from build123d import *

# Parameters (mm, degrees)
BOSS_EXTRUDE1_DEPTH = 0.7366
BOSS_EXTRUDE2_START = 5.3848
BOSS_EXTRUDE2_DEPTH = 0.7366
SKETCH2_R           = 1.1557
BOSS_EXTRUDE3_DEPTH = 4.6482
BOSS_EXTRUDE4_START = -5.3848
BOSS_EXTRUDE4_DEPTH = 0.7366
BOSS_EXTRUDE5_START = -6.1214
SKETCH2_2_R         = 1.1557
BOSS_EXTRUDE5_DEPTH = 4.6482


with BuildPart() as part:
    # Sketch1 → Boss-Extrude1 (new, symmetric)
    with BuildSketch(Plane.XY):
        with BuildLine():
            ThreePointArc((-1.5875, 2.421640582), (-6.0706, 0), (-1.5875, -2.421640582))
            ThreePointArc((-1.5875, -2.421640582), (0, -1.947681165), (1.5875, -2.421640582))
            ThreePointArc((1.5875, -2.421640582), (6.0706, 0), (1.5875, 2.421640582))
            ThreePointArc((1.5875, 2.421640582), (0, 1.947681165), (-1.5875, 2.421640582))
        make_face()
    extrude(amount=BOSS_EXTRUDE1_DEPTH, both=True)



with BuildPart() as body_2:
    # Sketch1<2> → Boss-Extrude2 (new body)
    with BuildSketch(Plane.XY.offset(BOSS_EXTRUDE2_START)):
        with BuildLine():
            ThreePointArc((-1.5875, 2.421640582), (-6.0706, 0), (-1.5875, -2.421640582))
            ThreePointArc((-1.5875, -2.421640582), (0, -1.947681165), (1.5875, -2.421640582))
            ThreePointArc((1.5875, -2.421640582), (6.0706, 0), (1.5875, 2.421640582))
            ThreePointArc((1.5875, 2.421640582), (0, 1.947681165), (-1.5875, 2.421640582))
        make_face()
    extrude(amount=BOSS_EXTRUDE2_DEPTH)


with BuildPart() as part_1:
    add(part.part)

    add(body_2.part)  # Boss-Extrude3 merges body 2
    # Sketch2 → Boss-Extrude3 (add)
    with BuildSketch(Plane.XY.offset(0.7366)):
        with Locations((-3.175, 0)):
            Circle(SKETCH2_R)
        with Locations((3.175, 0)):
            Circle(SKETCH2_R)
    extrude(amount=BOSS_EXTRUDE3_DEPTH)



with BuildPart() as body_2_2:
    # Sketch1<3> → Boss-Extrude4 (new body)
    with BuildSketch(Plane.XY.offset(BOSS_EXTRUDE4_START)):
        with BuildLine():
            ThreePointArc((-1.5875, 2.421640582), (-6.0706, 0), (-1.5875, -2.421640582))
            ThreePointArc((-1.5875, -2.421640582), (0, -1.947681165), (1.5875, -2.421640582))
            ThreePointArc((1.5875, -2.421640582), (6.0706, 0), (1.5875, 2.421640582))
            ThreePointArc((1.5875, 2.421640582), (0, 1.947681165), (-1.5875, 2.421640582))
        make_face()
    extrude(amount=-BOSS_EXTRUDE4_DEPTH)


with BuildPart() as part_2:
    add(part_1.part)

    add(body_2_2.part)  # Boss-Extrude5 merges body 2 2
    # Sketch2<2> → Boss-Extrude5 (add)
    with BuildSketch(Plane.XY.offset(0.7366).offset(BOSS_EXTRUDE5_START)):
        with Locations((-3.175, 0)):
            Circle(SKETCH2_2_R)
        with Locations((3.175, 0)):
            Circle(SKETCH2_2_R)
    extrude(amount=BOSS_EXTRUDE5_DEPTH)


solid = part_2.part
For this review, take the finished solid that the model builds, in its own axes (mm). A direction names the side the tool comes from. Round coordinates to 2 decimals unless told otherwise and drop trailing zeros. Loops run counter-clockwise (first coordinate to the right, second up) from the corner with the lowest first, then second, coordinate; pieces in that order, holes last. Notation, with made-up numbers: (-34, 74.25) - (-6, 74.25) arc R19 ccw to (-6, 96.25) - close; hole circle Ø3 at (-23, -21). An arc over 180 degrees is marked (long way). One line per question, with ' | ' between items.
Q1. The part is to be moulded in two halves that separate along X. For faces 1 (the flat face through (0, 0, -6.121)), 2 (the cylindrical face through (2.258, -0.703, 3.028)), say which applies: released by +X, released by -X, zero draft, split by the parting line, or undercut.
Taken from the geometry:
face 1: zero draft | face 2: undercut
Q2. For line 1 along Z through (x, y) = (-0.75, -1.7); line 2 along Y through (x, z) = (0, 0); line 3 along X through (y, z) = (-0.15, -3.75), list the stretches that pass through material, from the lowest coordinate up. Write a range as [from, to].
Taken from the geometry:
line 1: z = [-6.12, -5.38], [-0.74, 0.74], [5.38, 6.12] | line 2: y = [-1.95, 1.95] | line 3: x = [-4.32, -2.03], [2.03, 4.32]
Q3. Take a section at D-D (x = 4). Give the boundary of the cut face in (y, z).
Taken from the geometry:
outline: (-2.78, -6.12) - (2.78, -6.12) - (2.78, -5.38) - (0.81, -5.38) - (0.81, -0.74) - (2.78, -0.74) - (2.78, 0.74) - (0.81, 0.74) - (0.81, 5.38) - (2.78, 5.38) - (2.78, 6.12) - (-2.78, 6.12) - (-2.78, 5.38) - (-0.81, 5.38) - (-0.81, 0.74) - (-2.78, 0.74) - (-2.78, -0.74) - (-0.81, -0.74) - (-0.81, -5.38) - (-2.78, -5.38) - close
Q4. Take a section at A-A (y = 0). Give the boundary of the cut face in (x, z), and give its area (3 significant figures).
Taken from the geometry:
outline: (-6.07, -6.12) - (6.07, -6.12) - (6.07, -5.38) - (4.33, -5.38) - (4.33, -0.74) - (6.07, -0.74) - (6.07, 0.74) - (4.33, 0.74) - (4.33, 5.38) - (6.07, 5.38) - (6.07, 6.12) - (-6.07, 6.12) - (-6.07, 5.38) - (-4.33, 5.38) - (-4.33, 0.74) - (-6.07, 0.74) - (-6.07, -0.74) - (-4.33, -0.74) - (-4.33, -5.38) - (-6.07, -5.38) - close; hole (-2.02, -5.38) - (2.02, -5.38) - (2.02, -0.74) - (-2.02, -0.74) - close; hole (-2.02, 0.74) - (2.02, 0.74) - (2.02, 5.38) - (-2.02, 5.38) - close | area: 78.7 mm²
Q5. For pin 1 (1.5 mm diameter, centred on x = 3.5, z = 3.5, fed in from +Y); pin 2 (1.5 mm diameter, centred on x = 2, z = 2, fed in from +Y), all flat-tipped, find the tip position at first contact; note any pin that passes through.
Taken from the geometry:
pin 1: stops at y = 1.16 | pin 2: stops at y = 1.07
Q6. Tool access review of faces 3 (the flat face through (0, 0, 5.385)), 4 (the flat face through (0, 0, 6.121)): name each direction out of +Z, -Z, +X, -X, +Y, -Y from which nothing blocks a thin tool from reaching the whole face with its end or side.
Taken from the geometry:
face 3: none | face 4: +Z, +X, -X, +Y, -Y
Q7. Take a section at C-C (y = 1.45). Give the boundary of the cut face in (x, z).
Taken from the geometry:
outline: (-5.68, -6.12) - (5.68, -6.12) - (5.68, -5.38) - (-5.68, -5.38) - close; (-5.68, -0.74) - (5.68, -0.74) - (5.68, 0.74) - (-5.68, 0.74) - close; (-5.68, 5.38) - (5.68, 5.38) - (5.68, 6.12) - (-5.68, 6.12) - close
Q8. Take a section at B-B (z = -2.25). Give the boundary of the cut face in (x, y) (3 decimals), and give its area (3 significant figures).
Taken from the geometry:
outline: circle Ø2.311 at (-3.175, 0); circle Ø2.311 at (3.175, 0) | area: 8.39 mm²
